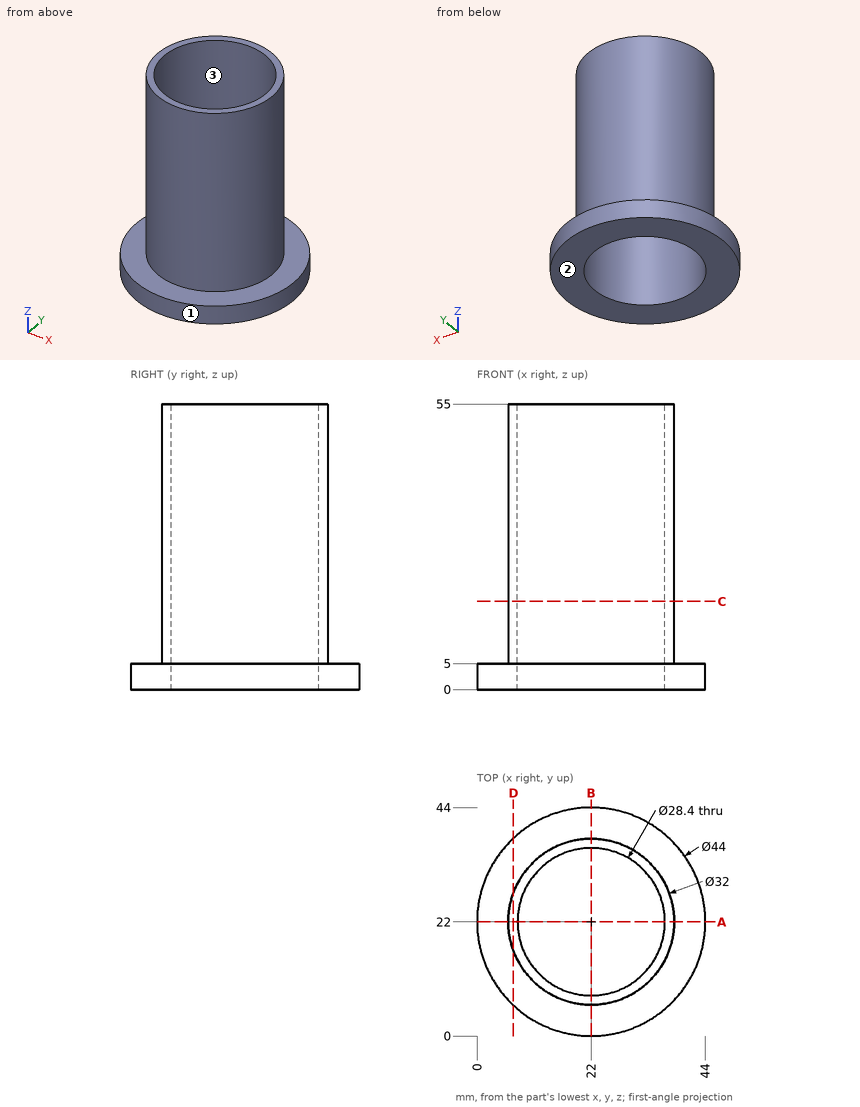
The drawing under review shows one solid part. Ordinate dimensions are in mm from its lowest x, y, z. Coordinates: 2 decimals unless noted, no trailing zeros. Write each loop counter-clockwise with the first axis right and the second up, starting at its lowest first coordinate (ties: lowest second). Pieces come first, ordered by that corner, then holes. Notation, with made-up numbers: (42.5, 23.5) - (62.5, 23.5) arc R22 cw to (62.5, 31.5) - close; hole circle Ø9 at (15.5, 56). An arc over 180 degrees is marked (long way). Use one line per item in the form item = value.
Q1. Consider section D-D (x = 7). Write out the cut boundary in (y, z), plus the area to 3 significant figures.
Taken from the geometry:
outline = (5.91, 0) - (38.09, 0) - (38.09, 5) - (27.57, 5) - (27.57, 55) - (16.43, 55) - (16.43, 5) - (5.91, 5) - close
area = 718 mm^2
Q2. Insertion check: pin 1 Ø10 at (x, z) = (13.5, 15) entering from +Y; pin 2 Ø4 at (y, z) = (16.5, 27) entering from +X; pin 3 Ø1.5 at (y, z) = (21.5, 13) entering from -X. Each pin has a flat end and moves straight along its axis. Give the tip position at first contact, or say it passes through.
Taken from the geometry:
pin_1 = 37.61
pin_2 = 37.61
pin_3 = 6
Q3. For probe 1 along Y at (x, z) = (22, 34); probe 2 along X at (y, z) = (22.5, 50.5); probe 3 along Z at (x, y) = (15, 42), list the stretches that pass through material, from the lowest coordinate up.
Taken from the geometry:
probe_1 = 6 to 7.8, 36.2 to 38
probe_2 = 6.01 to 7.81, 36.19 to 37.99
probe_3 = 0 to 5
Q4. Consider section C-C (z = 17). Write out the cut boundary in (x, y).
Taken from the geometry:
outline = circle Ø32 at (22, 22); hole circle Ø28.4 at (22, 22)
Q5. Consider section A-A (y = 22). Write out the cut boundary in (x, z).
Taken from the geometry:
outline = (0, 0) - (7.8, 0) - (7.8, 55) - (6, 55) - (6, 5) - (0, 5) - close; (36.2, 0) - (44, 0) - (44, 5) - (38, 5) - (38, 55) - (36.2, 55) - close
Q6. The part is to be moulded in two halves that separate along Y. For the marked faces 1, 2 and 3, say which applies: +Y half, -Y half, draft (parallel to the pull), parting line (faces both ways), or undercut.
Taken from the geometry:
face_1 = parting line
face_2 = draft
face_3 = undercut
